Work out the finished part from the listing and answer in its coordinate system (mm). Give positions to 0.01 mm unless a question says otherwise; leave off trailing zeros. Write each loop counter-clockwise with the first axis right and the second up, starting at its lowest first coordinate (ties: lowest second). Pieces come first, ordered by that corner, then holes. Notation, with made-up numbers: (34, 84) - (66, 84) arc R13 ccw to (66, 109) - close; hole circle Ø5 at (67, 78.5). An arc over 180 degrees is marked (long way). Write each question's results on one line, items separated by ' | '. Start each with the question number.
from build123d import *

# Parameters (mm, degrees)
BOSS_EXTRUDE1_DEPTH = 10
CUT_EXTRUDE1_REACH  = 56.851
SKETCH2_R           = 5.114059111


with BuildPart() as part:
    # Sketch1 → Boss-Extrude1 (new body)
    with BuildSketch(Plane.XY):
        with BuildLine():
            Line((0, 0), (-19.67027632, 0))
            Line((-19.67027632, 0), (-19.67027632, 40.381920209))
            ThreePointArc((-19.67027632, 40.381920209), (-9.83513816, 50.217058369), (0, 40.381920209))
            Line((0, 40.381920209), (0, 0))
        make_face()
    extrude(amount=BOSS_EXTRUDE1_DEPTH)

    # Sketch2 → Cut-Extrude1 (cut, up to next)
    with BuildSketch(Plane.XY.offset(10), mode=Mode.PRIVATE) as cut_extrude1_sk1:
        with Locations((-9.83513816, 40.381920209)):
            Circle(SKETCH2_R)
    cut_extrude1_tool1 = extrude(cut_extrude1_sk1.sketch, amount=-CUT_EXTRUDE1_REACH, mode=Mode.PRIVATE) & part.part
    add(cut_extrude1_tool1.solids().sort_by_distance((-9.835138, 40.38192, 10))[0], mode=Mode.SUBTRACT)


solid = part.part
Q1. A cutting plane is placed at A-A, the plane x = -8.5. Write down the section's boundary in (y, z).
Q2. Given pin 1 (8 mm diameter, centred on x = -9.84, y = 40.38, fed in from -Z), flat-ended and moving along its own axis, determine where the tip first touches the part or whether it passes through.
Q3. Consider L1, parallel to Y at x = -9.25, z = 5.75; L2, parallel to Y at x = -12, z = 7.25; L3, parallel to X at y = 44.5, z = 4.25. Determine where each line is inside the solid, lowest interval first.
Q4. A cutting plane is placed at D-D, the plane x = -1.25. Write down the section's boundary in (y, z), and give its area (3 significant figures).
Q5. The mould has two halves that part along Y. Classify faces 1 (the flat face through (-19.67, 20, 5)), 2 (the cylindrical face through (-10.051, 50.215, 4.93)), 3 (the cylindrical face through (-7.086, 44.694, 5.07)), 4 (the flat face through (-10, 0, 5)): pulls with the +Y half, pulls with the -Y half, needs draft (parallel to the pull), parting line crosses it, or undercut.
Q6. A cutting plane is placed at B-B, the plane y = 45. Write down the section's boundary in (x, z), and give its area (3 significant figures).
Result:
1) outline: (0, 0) - (35.45, 0) - (35.45, 10) - (0, 10) - close; (45.32, 0) - (50.13, 0) - (50.13, 10) - (45.32, 10) - close
2) pin 1: passes through
3) L1: y = 0 to 35.3, 45.46 to 50.2 | L2: y = 0 to 35.75, 45.02 to 49.98 | L3: x = -18.77 to -12.87, -6.8 to -0.9
4) outline: (0, 0) - (45.18, 0) - (45.18, 10) - (0, 10) - close | area: 452 mm2
5) face 1: needs draft | face 2: pulls with the +Y half | face 3: undercut | face 4: pulls with the -Y half
6) outline: (-18.52, 0) - (-12.03, 0) - (-12.03, 10) - (-18.52, 10) - close; (-7.64, 0) - (-1.15, 0) - (-1.15, 10) - (-7.64, 10) - close | area: 130 mm2
